Design review of the part built by this model. Coordinates are the model's own, in mm. A direction names the side the tool comes from. Round coordinates to 2 decimals unless told otherwise and drop trailing zeros. Loops run counter-clockwise (first coordinate to the right, second up) from the corner with the lowest first, then second, coordinate; pieces in that order, holes last. Notation, with made-up numbers: M 3,-38 L 18,-38 A10 ccw 18,-20 Z; hole C 19.25,56.5 d6. An arc over 180 degrees is marked long. Use a Markdown table: item, result.
Autodesk Inventor part; units mm, degrees
ref_plane "YZ Plane" through (0, 0, 0) normal (1, 0, 0) x (0, 1, 0)
ref_plane "XZ Plane" through (0, 0, 0) normal (0, 1, 0) x (-1, 0, 0)
ref_plane "XY Plane" through (0, 0, 0) normal (0, 0, 1) x (1, 0, 0)
sketch "Sketch1" plane through (0, 0, 0) normal (0, 0, 1) x (1, 0, 0)
  circle A0 centre (0, 0) radius 3.175
  circle A1 centre (0, 0) radius 12.7
  line L0 (-3.175, 12.2967) -> (3.175, 12.2967)
  line L1 (-3.175, 12.2967) -> (3.175, 12.2967)
  line L2 (3.175, 12.2967) -> (3.175, 24.9967)
  line L3 (3.175, 24.9967) -> (-3.175, 24.9967)
  line L4 (-3.175, 24.9967) -> (-3.175, 12.2967)
  dimension "d0" = 6.35
  dimension "d1" = 25.4
  dimension "d2" = 6.35
  dimension "d3" = 12.7
  dimension "d4" = 6.35
extrude "Extrusion1" add sketch "Sketch1" along normal blind 3.175
properties part number "spinnything"
1. Take a section at D-D on y = 18. Give the boundary of the cut face in (x, z) (3 decimals), and give its area (3 significant figures).
Check values:
| item | result |
|---|---|
| outline | M -3.175,0 L 3.175,0 L 3.175,3.175 L -3.175,3.175 Z |
| area | 20.2 mm² |
2. Take a section at A-A on x = 0. Give the boundary of the cut face in (y, z) (3 decimals), and give its area (3 significant figures).
Check values:
| item | result |
|---|---|
| outline | M -12.7,0 L -3.175,0 L -3.175,3.175 L -12.7,3.175 Z; M 3.175,0 L 24.997,0 L 24.997,3.175 L 3.175,3.175 Z |
| area | 99.5 mm² |
3. The part is to be moulded in two halves that separate along X. For faces 3 (the face through (0.51, -12.69, 1.57)), 4 (the face through (-0.69, 3.1, 1.57)), 5 (the face through (-3.175, 19, 2)), say which applies: pulls with the +X half, pulls with the -X half, needs draft (parallel to the pull), parting line crosses it, or undercut.
Check values:
| item | result |
|---|---|
| face 3 | parting line crosses it |
| face 4 | undercut |
| face 5 | pulls with the -X half |
4. Take a section at C-C on z = 2.7. Give the boundary of the cut face in (x, y) (3 decimals).
Check values:
| item | result |
|---|---|
| outline | M -3.175,12.297 A12.7 ccw long 3.175,12.297 L 3.175,24.997 L -3.175,24.997 Z; hole C 0,0 d6.35 |
5. Insertion check: pin 1 (1.6 mm diameter, centred on y = 18, z = 2, fed in from -X) (3 decimals); pin 2 (1.5 mm diameter, centred on x = -4.5, z = 2, fed in from +Y); pin 3 (1.6 mm diameter, centred on y = 17, z = 2, fed in from +X) (3 decimals). Each pin has a flat end and moves straight along its axis. Give the tip position at first contact, or say it passes through.
Check values:
| item | result |
|---|---|
| pin 1 | stops at x = -3.175 |
| pin 2 | stops at y = 12.13 |
| pin 3 | stops at x = 3.175 |
6. Take a section at B-B on y = 0. Give the boundary of the cut face in (x, z) (3 decimals).
Check values:
| item | result |
|---|---|
| outline | M -12.7,0 L -3.175,0 L -3.175,3.175 L -12.7,3.175 Z; M 3.175,0 L 12.7,0 L 12.7,3.175 L 3.175,3.175 Z |
7. Machinability: for faces 1 (the face through (0, 6, 0)), 2 (the face through (3.175, 19, 2)), which of the approach directions +Z, -Z, +X, -X, +Y, -Y give a long, thin tool a straight path to every point of the face, cutting with its end or side? Answer none if there is none.
Check values:
| item | result |
|---|---|
| face 1 | -Z, +X, -X, +Y, -Y |
| face 2 | +Z, -Z, +X, +Y |
8. Wall thickness on line 1 along Y through (x, z) = (0, 0.9) (3 decimals); line 2 along X through (y, z) = (18, 0.8) (3 decimals); line 3 along X through (y, z) = (-10, 2): over which ranges is each line inside the solid? List them lowest first. Write a range as from..to.
Check values:
| item | result |
|---|---|
| line 1 | y = -12.7..-3.175, 3.175..24.997 |
| line 2 | x = -3.175..3.175 |
| line 3 | x = -7.83..7.83 |
